from build123d import *

# Parameters (mm, degrees)
F0_R     = 1.6
F1_DEPTH = 2.75


with BuildPart() as f1:
    # F0 (on Top) → F1 (new body)
    with BuildSketch(Plane.XY):
        with BuildLine():
            ThreePointArc((-0.5, 0), (-1.671573, 2.828427), (-4.5, 4))
            ThreePointArc((-4.5, 4), (-8.5, -0.00086), (-4.49828, -4))
            ThreePointArc((-4.49828, -4), (-1.670965, -2.827819), (-0.5, 0))
        make_face()
        with Locations((-4.5, 0)):
            Circle(F0_R, mode=Mode.SUBTRACT)
        with BuildLine():
            ThreePointArc((4.5, -4), (0.5, 0), (4.5, 4))
            Line((4.5, 4), (-4.5, 4))
            ThreePointArc((-4.5, 4), (-1.671573, 2.828427), (-0.5, 0))
            ThreePointArc((-0.5, 0), (-1.670965, -2.827819), (-4.49828, -4))
            Line((-4.49828, -4), (4.5, -4))
        make_face()
        with BuildLine():
            ThreePointArc((4.5, -4), (7.328427, -2.828427), (8.5, 0))
            ThreePointArc((8.5, 0), (7.328427, 2.828427), (4.5, 4))
            ThreePointArc((4.5, 4), (0.5, 0), (4.5, -4))
        make_face()
        with Locations((4.5, 0)):
            Circle(F0_R, mode=Mode.SUBTRACT)
    extrude(amount=F1_DEPTH)


solid = f1.part
Could you check a few things on this model? Use its own coordinates, in mm. Round coordinates to 2 decimals unless told otherwise and drop trailing zeros. Order: outer loops, then holes, each group sorted by start corner. A loop starts at its lowest first (then second) coordinate and runs counter-clockwise, first axis right, second up. Notation, with made-up numbers: M -9,-18 L 6,-18 A30 cw 6,14 Z; hole C -25,18.25 d4. An arc over 180 degrees is marked long. One line per item, written item: value.
(1) Imagine slicing it at D-D (y = 1.25). Write out the boundary of the cut face in (x, z), and give its area (3 significant figures).
Ans:
outline: M -8.3,0 L -5.5,0 L -5.5,2.75 L -8.3,2.75 Z; M -3.5,0 L 3.5,0 L 3.5,2.75 L -3.5,2.75 Z; M 5.5,0 L 8.3,0 L 8.3,2.75 L 5.5,2.75 Z
area: 34.7 mm^2
(2) I'm going to push flat-ended pins straight in: P1, Ø1, axis at y = 1, z = 2.5, coming from the +X side; P2, Ø1, axis at y = -1.5, z = 0.5, coming from the -X side; P3, Ø3, axis at x = 4.5, y = 0, coming from the +Z side. Where does each tip first touch, or does it pass through?
Ans:
P1: stops at x = 8.47
P2: stops at x = -8.37
P3: passes through
(3) Imagine slicing it at A-A (z = 0.8). Write out the boundary of the cut face in (x, y), and give its area (3 significant figures).
Ans:
outline: M -4.5,-4 L 4.5,-4 A4 ccw 4.5,4 L -4.5,4 A4 ccw Z; hole C -4.5,0 d3.2; hole C 4.5,0 d3.2
area: 106 mm^2
(4) I need wall thicknesses on line 1 along Y through (x, z) = (-4.5, 0.85); line 2 along X through (y, z) = (0.5, 1.4); line 3 along X through (y, z) = (1.25, 0.9). Which ranges of each line are inside material? Lowest first, please. Write a range as from..to.
Ans:
line 1: y = -4..-1.6, 1.6..4
line 2: x = -8.47..-6.02, -2.98..2.98, 6.02..8.47
line 3: x = -8.3..-5.5, -3.5..3.5, 5.5..8.3
(5) Imagine slicing it at B-B (y = -0.25). Write out the boundary of the cut face in (x, z).
Ans:
outline: M -8.49,0 L -6.08,0 L -6.08,2.75 L -8.49,2.75 Z; M -2.92,0 L 2.92,0 L 2.92,2.75 L -2.92,2.75 Z; M 6.08,0 L 8.49,0 L 8.49,2.75 L 6.08,2.75 Z
(6) If we mould it in two halves opening along Y, with no side actions, what happens to faces 1 (the cylindrical face through (-8.5, 0.1, 1.4)), 2 (the cylindrical face through (-6.1, 0.07, 1.36)), 3 (the flat face through (0, 0, 2.75))? For each: released by +Y, released by -Y, zero draft, split by the parting line, or undercut.
Ans:
face 1: split by the parting line
face 2: undercut
face 3: zero draft
(7) Imagine slicing it at C-C (x = 3.25). Write out the boundary of the cut face in (y, z).
Ans:
outline: M -4,0 L -1,0 L -1,2.75 L -4,2.75 Z; M 1,0 L 4,0 L 4,2.75 L 1,2.75 Z
